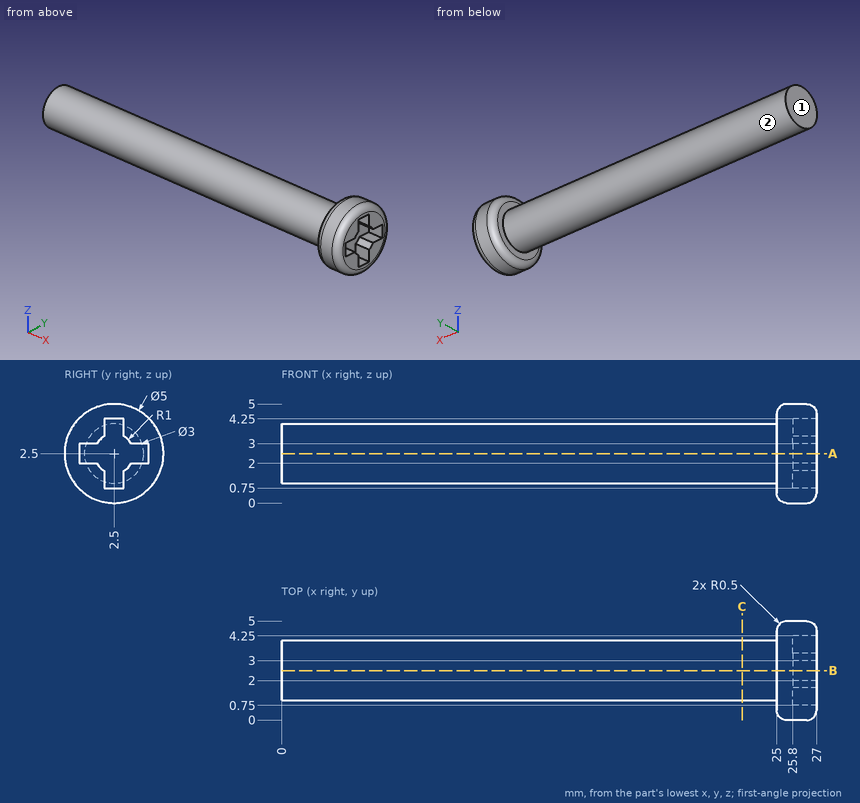
Here's the drawing with two shaded views (mm, measured from the low corner). I have some questions. A direction names the side the tool comes from. Give positions to 0.01 mm unless a question says otherwise; leave off trailing zeros. Order: outer loops, then holes, each group sorted by start corner. A loop starts at its lowest first (then second) coordinate and runs counter-clockwise, first axis right, second up. Notation, with made-up numbers: (-8.5, 32.5) - (35.5, 32.5) arc R9 cw to (35.5, 39.5) - close; hole circle Ø11 at (-18, 85.25). An arc over 180 degrees is marked (long way). Write each question's results on one line, items separated by ' | '.
1) Please list where these lines run through material, in increasing order: line 1 along X through (y, z) = (1.5, 4.05); line 2 along X through (y, z) = (2.3, 2.1); line 3 along Z through (x, y) = (12.25, 1.95). Write a range as [from, to].
Final values:
line 1: x = [25, 27] | line 2: x = [0, 25.8] | line 3: z = [1.1, 3.9]
2) Suppose I cut it at C-C, the plane x = 23.25. Write out the boundary of the cut face in (y, z).
Final values:
outline: circle Ø3 at (2.5, 2.5)
3) I'm going to push flat-ended pins straight in: pin 1 Ø1.5 at (x, z) = (13.5, 2) entering from -Y; pin 2 Ø0.7 at (x, z) = (26.5, 1.5) entering from -Y; pin 3 Ø1 at (x, z) = (26.5, 3.5) entering from +Y; pin 4 Ø2 at (y, z) = (3, 1.5) entering from -X. Where does each tip first touch, or does it pass through?
Final values:
pin 1: stops at y = 1 | pin 2: stops at y = 0.09 | pin 3: stops at y = 4.95 | pin 4: stops at x = 0
4) On a 3-axis mill with a long thin cutter (end or side, diameter ignored), from which of +Z, -Z, +X, -X, +Y, -Y can I reach the whole of each face in a straight line? I mean the marked faces 1 and 2. Say none if no direction works.
Final values:
face 1: +Z, -Z, -X, +Y, -Y | face 2: -X
5) Suppose I cut it at A-A, the plane z = 2.5. Write out the boundary of the cut face in (x, y), then the cut area to 3 significant figures.
Final values:
outline: (0, 1) - (25, 1) - (25, 0.5) arc R0.5 ccw to (25.5, 0) - (26.5, 0) arc R0.5 ccw to (27, 0.5) - (27, 0.75) - (25.8, 0.75) - (25.8, 4.25) - (27, 4.25) - (27, 4.5) arc R0.5 ccw to (26.5, 5) - (25.5, 5) arc R0.5 ccw to (25, 4.5) - (25, 4) - (0, 4) - close | area: 80.6 mm^2
